Part model, mm, in its own coordinate system. A direction names the side the tool comes from. Give positions to 0.01 mm unless a question says otherwise; leave off trailing zeros. Write each loop counter-clockwise with the first axis right and the second up, starting at its lowest first coordinate (ties: lowest second). Pieces come first, ordered by that corner, then holes.
```python
from build123d import *

# Parameters (mm, degrees)
SKETCH_W      = 25
SKETCH_H      = 25
SKETCH_R      = 1.8
SKETCH_R_2    = 4
PAD_DEPTH     = 3
SKETCH001_R   = 7.5
SKETCH001_R_2 = 4
PAD001_DEPTH  = 21


with BuildPart() as part:
    # Sketch → Pad (new body)
    with BuildSketch(Plane.XY):
        Rectangle(SKETCH_W, SKETCH_H)
        with Locations((-8.485281, 8.485281)):
            Circle(SKETCH_R, mode=Mode.SUBTRACT)
        with Locations((8.485281, 8.485281)):
            Circle(SKETCH_R, mode=Mode.SUBTRACT)
        with Locations((-8.485281, -8.485281)):
            Circle(SKETCH_R, mode=Mode.SUBTRACT)
        with Locations((8.485281, -8.485281)):
            Circle(SKETCH_R, mode=Mode.SUBTRACT)
        Circle(SKETCH_R_2, mode=Mode.SUBTRACT)
    extrude(amount=PAD_DEPTH)

    # Sketch001 → Pad001 (new body)
    with BuildSketch(Plane.XY.offset(3)):
        Circle(SKETCH001_R)
        Circle(SKETCH001_R_2, mode=Mode.SUBTRACT)
    extrude(amount=PAD001_DEPTH)


solid = part.part
```
1) Wall check: L1, parallel to Y at x = 0, z = 13.75; L2, parallel to Z at x = 6.25, y = -9; L3, parallel to Y at x = -2.25, z = 9.5. Give the ranges that are in metal, low to high.
Answers follow:
L1: y = -7.5 to -4, 4 to 7.5
L2: z = 0 to 3
L3: y = -7.15 to -3.31, 3.31 to 7.15
2) Two-plate mould, pull along Y, no slides. Class faces 1 (the face through (0, 12.5, 1)), 2 (the face through (9.453, 10.003, 1.479)), 3 (the face through (3, -3, 24)): +Y half, -Y half, draft (parallel to the pull), parting line (faces both ways), or undercut.
Answers follow:
face 1: +Y half
face 2: undercut
face 3: draft
3) Pin check, flat tips, straight feed: pin 1 Ø2 at (x, y) = (8.49, -8.49) entering from +Z; pin 2 Ø6 at (y, z) = (-2, 16) entering from -X; pin 3 Ø4 at (x, y) = (-8.49, -8.49) entering from +Z; pin 4 Ø6 at (x, z) = (4, 14.5) entering from +Y. Stop position of each tip, or through.
Answers follow:
pin 1: passes through
pin 2: stops at x = -7.5
pin 3: stops at z = 3
pin 4: stops at y = 7.43
4) Saw through at C-C, the plane y = 6. Write the cut outline in (x, z).
Answers follow:
outline: (-12.5, 0) - (12.5, 0) - (12.5, 3) - (4.5, 3) - (4.5, 24) - (-4.5, 24) - (-4.5, 3) - (-12.5, 3) - close
5) Saw through at D-D, the plane x = 8.25. Write the cut outline in (y, z), then the cut area to 3 significant figures.
Answers follow:
outline: (-12.5, 0) - (-10.27, 0) - (-10.27, 3) - (-12.5, 3) - close; (-6.7, 0) - (6.7, 0) - (6.7, 3) - (-6.7, 3) - close; (10.27, 0) - (12.5, 0) - (12.5, 3) - (10.27, 3) - close
area: 53.6 mm2
6) 3-axis set-ups, long thin cutter, end or side, ignore diameter. For faces 4 (the face through (-6, 6, 3)), 5 (the face through (9.32, -10.08, 1.48)): which of +Z, -Z, +X, -X, +Y, -Y reach the whole face in a straight line?
Answers follow:
face 4: +Z
face 5: +Z, -Z
7) Saw through at A-A, the plane y = 0. Write the cut outline in (x, z).
Answers follow:
outline: (-12.5, 0) - (-4, 0) - (-4, 24) - (-7.5, 24) - (-7.5, 3) - (-12.5, 3) - close; (4, 0) - (12.5, 0) - (12.5, 3) - (7.5, 3) - (7.5, 24) - (4, 24) - close
